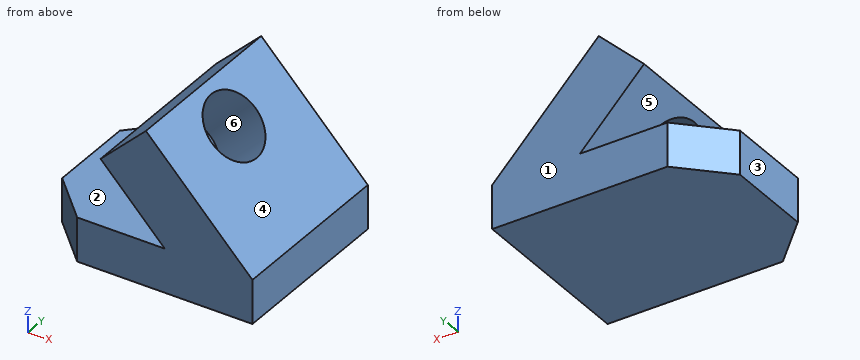
```python
from build123d import *

# Parameters (mm, degrees)
F1_DEPTH = 25.4
F3_W     = 203.2
F3_H     = 177.8
F3_R     = 38.1
F5_DEPTH = 73.084924


with BuildPart() as f1:
    # F0 (on Top) → F1 (new body, symmetric)
    with BuildSketch(Plane.XY):
        Polygon((-50.8, 50.8), (0, 0), (203.2, 0), (203.2, 203.2), (0, 203.2), (-50.8, 152.4), align=None)
    extrude(amount=F1_DEPTH, both=True)

    # F3 (on face) → F5 (join, through all)
    with BuildSketch(Plane(origin=(117.838052, 0, 113.794884), x_dir=(0, 1, 0), z_dir=(0.71934, 0, 0.694658))):
        with Locations((101.6, -33.98335)):
            Rectangle(F3_W, F3_H)
        with Locations((101.6, 4.11665)):
            Circle(F3_R, mode=Mode.SUBTRACT)
    extrude(amount=-F5_DEPTH)


solid = f1.part
```
Build history of the part. All positions in model axes, mm. Face numbers are marked on the shaded views. A direction names the side the tool comes from. Round coordinates to 2 decimals unless told otherwise and drop trailing zeros. Write each loop counter-clockwise with the first axis right and the second up, starting at its lowest first coordinate (ties: lowest second). Pieces come first, ordered by that corner, then holes.
1) Band-saw the part on D-D, the plane x = -7. List the corners of the cut face in (y, z).
2) Band-saw the part on C-C, the plane z = -10.5. List the corners of the cut face in (x, y).
3) Mould opens along Z. For the marked faces 3, 4, 5 and 6 say: +Z half, -Z half, draft (parallel to the pull), parting line (faces both ways), or undercut.
4) Drill centre lines: probe 1 along Z at (x, y) = (-16, 111); probe 2 along Z at (x, y) = (79.5, 16); probe 3 along Z at (x, y) = (77, 29.5). Where is each one in solid material? Low to high.
5) 3-axis set-ups, long thin cutter, end or side, ignore diameter. For the marked faces 1 and 2: which of +Z, -Z, +X, -X, +Y, -Y reach the whole face in a straight line?
6) Pin check, flat tips, straight feed: pin 1 (10 mm diameter, centred on y = 83.5, z = 38, fed in from +X); pin 2 (5 mm diameter, centred on y = 58, z = 128, fed in from +X); pin 3 (3 mm diameter, centred on y = 44, z = 105.5, fed in from +X). Stop position of each tip, or through.
Ans:
1. outline: (7, -25.4) - (196.2, -25.4) - (196.2, 25.4) - (7, 25.4) - close
2. outline: (-50.8, 50.8) - (0, 0) - (203.2, 0) - (203.2, 203.2) - (0, 203.2) - (-50.8, 152.4) - close
3. face 3: draft
3. face 4: +Z half
3. face 5: undercut
3. face 6: undercut
4. probe 1: z = -25.4 to 25.4
4. probe 2: z = -25.4 to 25.4, 48.29 to 153.12
4. probe 3: z = -25.4 to 25.4, 50.87 to 150.7
5. face 1: +Z, -Z, +X, -X, +Y
5. face 2: -X, +Y, -Y
6. pin 1: stops at x = 195.86
6. pin 2: stops at x = 106.53
6. pin 3: stops at x = 127.3
